from build123d import *

# Parameters (mm, degrees)
SKETCH1_W              = 13
SKETCH1_H              = 188.148975749
BOSS_EXTRUDE1_DEPTH    = 8
SKETCH2_W              = 45
SKETCH2_H              = 52
CUT_EXTRUDE1_DEPTH     = 341.17998495
SPLIT1_SURFACE_1_BACK  = 341.18
SPLIT1_SURFACE_1_DEPTH = 682.36
SPLIT1_SURFACE_2_BACK  = 341.18
SPLIT1_SURFACE_2_DEPTH = 682.36
SKETCH5_R              = 2.5
CUT_EXTRUDE6_DEPTH     = 5.2
CUT_EXTRUDE7_START     = -5.2
SKETCH4_R              = 2.5
CUT_EXTRUDE7_DEPTH     = 5.2


with BuildPart() as part:
    # Sketch1 → Boss-Extrude1 (new body)
    with BuildSketch(Plane.XY):
        with BuildLine():
            Line((0, 30.859943174), (0, 219.008918923))
            ThreePointArc((0, 219.008918923), (0.311003468, 220.744808182), (1.205324608, 222.264750409))
            Line((1.205324608, 222.264750409), (42.261389271, 270.115641625))
            ThreePointArc((42.261389271, 270.115641625), (42.81710491, 270.906904614), (43.210130369, 271.790334282))
            Line((43.210130369, 271.790334282), (54.802396658, 306.567133147))
            ThreePointArc((54.802396658, 306.567133147), (56.605292439, 309.029920375), (59.503914938, 309.985818768))
            Line((59.503914938, 309.985818768), (80.378944352, 309.985818768))
            ThreePointArc((80.378944352, 309.985818768), (83.277566851, 309.029920375), (85.080462632, 306.567133147))
            Line((85.080462632, 306.567133147), (96.672728921, 271.790334282))
            ThreePointArc((96.672728921, 271.790334282), (97.06575438, 270.906904614), (97.621470019, 270.115641625))
            Line((97.621470019, 270.115641625), (138.677534682, 222.264750409))
            ThreePointArc((138.677534682, 222.264750409), (139.571855822, 220.744808182), (139.88285929, 219.008918923))
            Line((139.88285929, 219.008918923), (139.88285929, 30.859943174))
            ThreePointArc((139.88285929, 30.859943174), (138.418393196, 27.324409268), (134.88285929, 25.859943174))
            Line((134.88285929, 25.859943174), (117.446021446, 25.859943174))
            ThreePointArc((117.446021446, 25.859943174), (115.538843756, 25.481920377), (113.920048724, 24.405012478))
            Line((113.920048724, 24.405012478), (89.38285929, 0))
            Line((89.38285929, 0), (50.5, 0))
            Line((50.5, 0), (25.962810565, 24.405012478))
            ThreePointArc((25.962810565, 24.405012478), (24.344015534, 25.481920377), (22.436837844, 25.859943174))
            Line((22.436837844, 25.859943174), (5, 25.859943174))
            ThreePointArc((5, 25.859943174), (1.464466094, 27.324409268), (0, 30.859943174))
        make_face()
        with Locations((19.5, 124.934431049)):
            Rectangle(SKETCH1_W, SKETCH1_H, mode=Mode.SUBTRACT)
        with Locations((120.5, 124.934431049)):
            Rectangle(SKETCH1_W, SKETCH1_H, mode=Mode.SUBTRACT)
    extrude(amount=BOSS_EXTRUDE1_DEPTH)

    # Sketch2 → Cut-Extrude1 (cut, through all)
    with BuildSketch(Plane.XY.offset(8)):
        with Locations((69.88285929, 180.008918923)):
            Rectangle(SKETCH2_W, SKETCH2_H)
    extrude(amount=-CUT_EXTRUDE1_DEPTH, mode=Mode.SUBTRACT)


with BuildPart() as body_2:
    # Split1: the piece behind the surface
    add(part.part)
    # Split1 surface: a surface, the sketch's curves swept straight by 682.36 mm
    with BuildLine(Plane(origin=(0, 0, 0), x_dir=(-1, 0, 0), z_dir=(0, 0, -1)).offset(-SPLIT1_SURFACE_1_BACK), mode=Mode.PRIVATE) as split1_surface_1_path:
        Line((0, 115.359943174), (-139.88285929, 115.359943174))
    split1_surface_1 = Shell.extrude(split1_surface_1_path.wire(), (0 * SPLIT1_SURFACE_1_DEPTH, 0 * SPLIT1_SURFACE_1_DEPTH, -1 * SPLIT1_SURFACE_1_DEPTH))
    split(bisect_by=split1_surface_1, keep=Keep.BOTTOM)


with BuildPart() as part_1:
    add(part.part)

    # Split1: split by a surface, the side it looks to stays
    # Split1 surface: a surface, the sketch's curves swept straight by 682.36 mm
    with BuildLine(Plane(origin=(0, 0, 0), x_dir=(-1, 0, 0), z_dir=(0, 0, -1)).offset(-SPLIT1_SURFACE_2_BACK), mode=Mode.PRIVATE) as split1_surface_2_path:
        Line((0, 115.359943174), (-139.88285929, 115.359943174))
    split1_surface_2 = Shell.extrude(split1_surface_2_path.wire(), (0 * SPLIT1_SURFACE_2_DEPTH, 0 * SPLIT1_SURFACE_2_DEPTH, -1 * SPLIT1_SURFACE_2_DEPTH))
    split(bisect_by=split1_surface_2, keep=Keep.TOP)

    # Sketch5 → Cut-Extrude6 (cut)
    with BuildSketch(Plane(origin=(0, 115.359943174, -115.359943174), x_dir=(1, 0, 0), z_dir=(0, -1, 0))):
        with Locations(Location((133.441429645, 119.359943174, 0), (0, 0, 270))):
            Circle(SKETCH5_R)
        with Locations(Location((70, 119.359943174, 0), (0, 0, 270))):
            Circle(SKETCH5_R)
        with Locations(Location((100, 119.359943174, 0), (0, 0, 270))):
            Circle(SKETCH5_R)
        with Locations(Location((40, 119.359943174, 0), (0, 0, 270))):
            Circle(SKETCH5_R)
        with Locations(Location((6.5, 119.359943174, 0), (0, 0, 270))):
            Circle(SKETCH5_R)
    extrude(amount=CUT_EXTRUDE6_DEPTH, mode=Mode.SUBTRACT)


with BuildPart() as body_2_1:
    # Body-Move/Copy1: moved
    add(body_2.part.moved(Location((0, 34.793425009, 0))))

    # Sketch4 → Cut-Extrude7 (cut)
    with BuildSketch(Plane(origin=(0, 150.153368183, 0), x_dir=(-1, 0, 0), z_dir=(0, -1, 0)).offset(CUT_EXTRUDE7_START)):
        with Locations(Location((-6.5, -4, 0), (0, 0, 90))):
            Circle(SKETCH4_R)
        with Locations(Location((-70, -4, 0), (0, 0, 90))):
            Circle(SKETCH4_R)
        with Locations(Location((-40, -4, 0), (0, 0, 90))):
            Circle(SKETCH4_R)
        with Locations(Location((-100, -4, 0), (0, 0, 90))):
            Circle(SKETCH4_R)
        with Locations(Location((-133.441429645, -4, 0), (0, 0, 90))):
            Circle(SKETCH4_R)
    extrude(amount=CUT_EXTRUDE7_DEPTH, mode=Mode.SUBTRACT)


solid = part_1.part
Check sheet for the modelled part. Datum: model origin and axes. Units: mm. A direction names the side the tool comes from. Coordinates: 2 decimals unless noted, no trailing zeros. Loops run counter-clockwise (first coordinate to the right, second up) from the corner with the lowest first, then second, coordinate; pieces in that order, holes last. Notation, with made-up numbers: (43, 89.5) -> (86, 89.5) arc R26 ccw to (86, 125.5) -> close; hole circle Ø7 at (1, 57). An arc over 180 degrees is marked (long way). Answer in a Markdown table with one row per item.
1. Sectioned sample at A-A, the plane y = 41.5. Record the boundary of the cut face in (x, z), then the cut area to 3 significant figures.
Check values:
| item | result |
|---|---|
| outline | (0, 0) -> (13, 0) -> (13, 8) -> (0, 8) -> close; (26, 0) -> (114, 0) -> (114, 8) -> (26, 8) -> close; (127, 0) -> (139.88, 0) -> (139.88, 8) -> (127, 8) -> close |
| area | 911 mm2 |
2. Go/stop test with flat-tipped pins: pin 1 (3 mm diameter, centred on x = 133.44, z = 4, fed in from -Y); pin 2 (2.5 mm diameter, centred on x = 69.5, z = 4, fed in from +Y); pin 3 (1.5 mm diameter, centred on y = 15.5, z = 3.5, fed in from +X). Record where each tip stops, or that it passes through.
Check values:
| item | result |
|---|---|
| pin 1 | stops at y = 25.86 |
| pin 2 | stops at y = 110.16 |
| pin 3 | stops at x = 105.72 |
3. Release check for a two-part mould opening along Z. For faces 6 (the face through (133, 110.16, 4)), 7 (the face through (13, 73, 4)) record: released by +Z, released by -Z, zero draft, split by the parting line, or undercut.
Check values:
| item | result |
|---|---|
| face 6 | undercut |
| face 7 | zero draft |
4. Sectioned sample at C-C, the plane x = 6.5. Record the boundary of the cut face in (y, z).
Check values:
| item | result |
|---|---|
| outline | (25.86, 0) -> (115.36, 0) -> (115.36, 1.5) -> (110.16, 1.5) -> (110.16, 6.5) -> (115.36, 6.5) -> (115.36, 8) -> (25.86, 8) -> close |
5. Material ranges on line 1 along X through (y, z) = (51, 3.25); line 2 along Y through (x, z) = (122, 5.5); line 3 along Z through (x, y) = (6, 111), recorded low to high. Write a range as [from, to].
Check values:
| item | result |
|---|---|
| line 1 | x = [0, 13], [26, 114], [127, 139.88] |
| line 2 | y = [25.86, 30.86] |
| line 3 | z = [0, 1.55], [6.45, 8] |
6. Sectioned sample at D-D, the plane x = 95. Record the boundary of the cut face in (y, z), then the cut area to 3 significant figures.
Check values:
| item | result |
|---|---|
| outline | (5.59, 0) -> (115.36, 0) -> (115.36, 8) -> (5.59, 8) -> close |
| area | 878 mm2 |
7. Access from +Z, -Z, +X, -X, +Y, -Y to the whole of each face (thin tool, end or side, straight path). Record for faces 1 (the face through (139.883, 74, 4)), 2 (the face through (26, 73, 4)), 3 (the face through (40, 110.16, 4)), 4 (the face through (0, 73, 4)), 5 (the face through (126, 25.86, 4)).
Check values:
| item | result |
|---|---|
| face 1 | +Z, -Z, +X, +Y, -Y |
| face 2 | +Z, -Z, +Y |
| face 3 | +Y |
| face 4 | +Z, -Z, -X, +Y, -Y |
| face 5 | +Z, -Z, +X, -Y |
8. Sectioned sample at B-B, the plane x = 70. Record the boundary of the cut face in (y, z).
Check values:
| item | result |
|---|---|
| outline | (0, 0) -> (115.36, 0) -> (115.36, 1.5) -> (110.16, 1.5) -> (110.16, 6.5) -> (115.36, 6.5) -> (115.36, 8) -> (0, 8) -> close |
